```python
from build123d import *

# Parameters (mm, degrees)
SKETCH1_R           = 16.5
SKETCH1_R_2         = 9.5
SKETCH1_R_3         = 1.75
BOSS_EXTRUDE1_DEPTH = 6
SKETCH2_R           = 2.8
CUT_EXTRUDE1_DEPTH  = 3
BOSS_EXTRUDE2_START = -5
SKETCH3_R           = 20
SKETCH3_R_2         = 1.75
SKETCH3_R_3         = 2.8
BOSS_EXTRUDE2_DEPTH = 5
SKETCH6_R           = 2.55
CUT_EXTRUDE3_DEPTH  = 5
SKETCH7_R           = 10
CUT_EXTRUDE4_DEPTH  = 29.91366459
FILLET1_R           = 0.2
CHAMFER1_SIZE       = 0.5


with BuildPart() as part:
    # Sketch1 → Boss-Extrude1 (new body)
    with BuildSketch(Plane.XY):
        Circle(SKETCH1_R)
        Circle(SKETCH1_R_2, mode=Mode.SUBTRACT)
        with Locations((12.5, 0)):
            Circle(SKETCH1_R_3, mode=Mode.SUBTRACT)
        with Locations((0, -12.5)):
            Circle(SKETCH1_R_3, mode=Mode.SUBTRACT)
        with Locations((-12.5, 0)):
            Circle(SKETCH1_R_3, mode=Mode.SUBTRACT)
        with Locations((0, 12.5)):
            Circle(SKETCH1_R_3, mode=Mode.SUBTRACT)
    extrude(amount=BOSS_EXTRUDE1_DEPTH)

    # Sketch2 → Cut-Extrude1 (cut)
    with BuildSketch(Plane.XY.offset(6)):
        with Locations((12.5, 0)):
            Circle(SKETCH2_R)
    extrude(amount=-CUT_EXTRUDE1_DEPTH, mode=Mode.SUBTRACT)

    # Sketch3 → Boss-Extrude2 (add)
    with BuildSketch(Plane.XY.offset(6).offset(BOSS_EXTRUDE2_START)):
        Circle(SKETCH3_R)
        with Locations((12.5, 0)):
            Circle(SKETCH3_R_2, mode=Mode.SUBTRACT)
        with Locations((0, -12.5)):
            Circle(SKETCH3_R_3, mode=Mode.SUBTRACT)
        with Locations((-12.5, 0)):
            Circle(SKETCH3_R_3, mode=Mode.SUBTRACT)
        with Locations((0, 12.5)):
            Circle(SKETCH3_R_3, mode=Mode.SUBTRACT)
    extrude(amount=BOSS_EXTRUDE2_DEPTH)

    # Sketch6 → Cut-Extrude3 (cut)
    with BuildSketch(Plane.XY.offset(6)):
        with Locations((-10.606601718, -10.606601718)):
            Circle(SKETCH6_R)
    extrude(amount=-CUT_EXTRUDE3_DEPTH, mode=Mode.SUBTRACT)

    # Sketch7 → Cut-Extrude4 (cut, through all)
    with BuildSketch(Plane.XY.offset(6)):
        Circle(SKETCH7_R)
    extrude(amount=-CUT_EXTRUDE4_DEPTH, mode=Mode.SUBTRACT)

    # Fillet1
    fillet1_edges = [part.edges().sort_by_distance(p)[0] for p in [
        (-10, 0, 0),
        (-10, 0, 6),
    ]]
    fillet(fillet1_edges, radius=FILLET1_R)

    # Chamfer1
    chamfer1_edges = [part.edges().sort_by_distance(p)[0] for p in [
        (-20, 0, 6),
        (-20, 0, 1),
    ]]
    chamfer(chamfer1_edges, length=CHAMFER1_SIZE)


solid = part.part
```
The model under review builds one solid part; all positions refer to its coordinate system, in mm. A direction names the side the tool comes from. Round coordinates to 2 decimals unless told otherwise and drop trailing zeros. Loops run counter-clockwise (first coordinate to the right, second up) from the corner with the lowest first, then second, coordinate; pieces in that order, holes last. Notation, with made-up numbers: M -39.5,-16.75 L 5.5,-16.75 A24 ccw 5.5,2.25 Z; hole C 34.5,18.5 d6. An arc over 180 degrees is marked long. Write item = value, one per line.
Item 1: The part is to be moulded in two halves that separate along Y. For faces 4 (the flat face through (-10, -11, 1)), 5 (the cylindrical face through (15.24, -6.32, 0.49)), 6 (the flat face through (8, -8, 6)), say which applies: released by +Y, released by -Y, zero draft, split by the parting line, or undercut.
Return value:
face_4 = undercut
face_5 = split by the parting line
face_6 = zero draft
Item 2: Insertion check: P1, Ø3, axis at x = -7, z = 4.5, coming from the +Y side; P2, Ø3, axis at y = -12, z = 1.5, coming from the -X side; P3, Ø1.5, axis at x = -10.5, y = -11, coming from the +Z side; P4, Ø3, axis at x = 0, y = -12.5, coming from the -Z side. Each pin has a flat end and moves straight along its axis. Give the tip position at first contact, or say it passes through.
Return value:
P1 = 19.23
P2 = -17.02
P3 = 1
P4 = through
Item 3: Take a section at D-D on x = -12.5. State how many separate pieces and enclosed holes the cut face has, then the cut area to 3 significant figures.
Return value:
separate_pieces = 3
enclosed_holes = 0
area = 139 mm2
Item 4: Take a section at C-C on z = 2.4. Write out the cut boundary in (x, y), then the cut area to 3 significant figures.
Return value:
outline = C 0,0 d40; hole C -12.5,0 d3.5; hole C -10.61,-10.61 d5.1; hole C 0,0 d20; hole C 0,-12.5 d3.5; hole C 0,12.5 d3.5; hole C 12.5,0 d3.5
area = 884 mm2
Item 5: Machinability: for faces 1 (the flat face through (-8.8, -14.4, 1)), 2 (the cylindrical face through (-8.25, -11.58, 3.54)), 3 (the cylindrical face through (-0.228, -10.765, 2.958)), which of the approach directions +Z, -Z, +X, -X, +Y, -Y give a long, thin tool a straight path to every point of the face, cutting with its end or side? Answer none if there is none.
Return value:
face_1 = -Z
face_2 = +Z
face_3 = +Z, -Z
Item 6: Take a section at A-A on y = 0. Write out the cut boundary in (x, z).
Return value:
outline = M -20,1.5 L -19.5,1 L -16.5,1 L -16.5,0 L -14.25,0 L -14.25,6 L -19.5,6 L -20,5.5 Z; M -10.75,0 L -10.2,0 A0.2 ccw -10,0.2 L -10,5.8 A0.2 ccw -10.2,6 L -10.75,6 Z; M 10,0.2 A0.2 ccw 10.2,0 L 10.75,0 L 10.75,6 L 10.2,6 A0.2 ccw 10,5.8 Z; M 14.25,0 L 16.5,0 L 16.5,1 L 19.5,1 L 20,1.5 L 20,5.5 L 19.5,6 L 14.25,6 Z
Item 7: For line 1 (Y direction, x = 0, z = 4.3); line 2 (Z direction, x = 16.5, y = -4); line 3 (X direction, y = 2.5, z = 1.15), list the stretches that pass through material, from the lowest coordinate up. Write a range as [from, to].
Return value:
line_1 = [-20, -14.25], [-10.75, -10], [10, 10.75], [14.25, 20]
line_2 = [1, 6]
line_3 = [-19.49, -9.68], [9.68, 19.49]
